```python
from build123d import *

# Parameters (mm, degrees)
SKETCH_1_W      = 84.65
SKETCH_1_H      = 48
SKETCH_1_R      = 1.5
EXTRUDE_1_DEPTH = 1.63
FILLET_1_R      = 3
SKETCH_4_W      = 7.5
SKETCH_4_H      = 8.6
EXTRUDE_2_DEPTH = 27.44
EXTRUDE_3_DEPTH = 16


with BuildPart() as part:
    # 草图1 → 凸台-拉伸1 (new body)
    with BuildSketch(Plane(origin=(0, 0, 0), x_dir=(1, 0, 0), z_dir=(0, 1, 0))):
        with Locations((42.325, 24)):
            Rectangle(SKETCH_1_W, SKETCH_1_H)
        with Locations(Location((2.9, 45, 0), (0, 0, 270))):
            Circle(SKETCH_1_R, mode=Mode.SUBTRACT)
        with Locations(Location((2.9, 13.3, 0), (0, 0, 270))):
            Circle(SKETCH_1_R, mode=Mode.SUBTRACT)
        with Locations(Location((82.15, 45, 0), (0, 0, 270))):
            Circle(SKETCH_1_R, mode=Mode.SUBTRACT)
        with Locations(Location((82.15, 13.3, 0), (0, 0, 270))):
            Circle(SKETCH_1_R, mode=Mode.SUBTRACT)
    extrude(amount=EXTRUDE_1_DEPTH)

    # 圆角1
    fillet_1_edges = [part.edges().sort_by_distance(p)[0] for p in [
        (0, 0.815, 0),
        (0, 0.815, -48),
        (84.65, 0.815, -48),
        (84.65, 0.815, 0),
    ]]
    fillet(fillet_1_edges, radius=FILLET_1_R)

    # 草图4 → 凸台-拉伸2 (add)
    with BuildSketch(Plane(origin=(51.65, 0, 0), x_dir=(0, 0, -1), z_dir=(1, 0, 0))):
        with Locations((3.75, 5.93)):
            Rectangle(SKETCH_4_W, SKETCH_4_H)
    extrude(amount=EXTRUDE_2_DEPTH)

    # 草图5 → 凸台-拉伸3 (add)
    with BuildSketch(Plane(origin=(0, 1.63, 0), x_dir=(1, 0, 0), z_dir=(0, 1, 0))):
        Polygon((62.31, 29.58), (62.31, 16.3), (59.81, 13.98), (58.31, 13.98), (56.81, 13.98), (54.31, 16.3), (54.31, 29.58), align=None)
        Polygon((10.31, 13.98), (8.81, 13.98), (6.31, 16.3), (6.31, 29.58), (14.31, 29.58), (14.31, 16.3), (11.81, 13.98), align=None)
    extrude(amount=EXTRUDE_3_DEPTH)


solid = part.part
```
Build history of the part. All positions in model axes, mm. A direction names the side the tool comes from. Coordinates: 2 decimals unless noted, no trailing zeros. Order: outer loops, then holes, each group sorted by start corner. A loop starts at its lowest first (then second) coordinate and runs counter-clockwise, first axis right, second up.
Item 1: Mould opens along X. For faces 5 (the flat face through (7.58, 9.52, -15.12)), 6 (the flat face through (13.08, 9.52, -15.16)), 7 (the flat face through (10, 10, -13.98)), 8 (the flat face through (61.08, 9.52, -15.16)) say: released by +X, released by -X, zero draft, split by the parting line, or undercut.
Filled in:
face 5: released by -X
face 6: undercut
face 7: zero draft
face 8: released by +X
Item 2: Tool access for faces 1 (the flat face through (6.31, 10, -23)), 2 (the flat face through (14.31, 10, -23)), 3 (the flat face through (65, 6, -7.5)), 4 (the flat face through (54.31, 10, -23)): list every direction of +Z, -Z, +X, -X, +Y, -Y with a clear straight run to the whole face (end or side of a thin tool).
Filled in:
face 1: +Z, -Z, -X, +Y
face 2: +Z, -Z, +Y
face 3: +X, -X, +Y
face 4: -Z, +Y
Item 3: Saw through at A-A on y = 6. List the corners of the cut face in (x, z), then the cut area to 3 significant figures.
Filled in:
outline: (6.31, -29.58) - (14.31, -29.58) - (14.31, -16.3) - (11.81, -13.98) - (8.81, -13.98) - (6.31, -16.3) - close; (51.65, -7.5) - (79.09, -7.5) - (79.09, 0) - (51.65, 0) - close; (54.31, -29.58) - (62.31, -29.58) - (62.31, -16.3) - (59.81, -13.98) - (56.81, -13.98) - (54.31, -16.3) - close
area: 444 mm2
Item 4: Saw through at C-C on x = 65. List the corners of the cut face in (y, z), then the cut area to 3 significant figures.
Filled in:
outline: (0, -48) - (1.63, -48) - (1.63, -7.5) - (10.23, -7.5) - (10.23, 0) - (0, 0) - close
area: 143 mm2
Item 5: Saw through at B-B on y = 13.75. List the corners of the cut face in (x, z).
Filled in:
outline: (6.31, -29.58) - (14.31, -29.58) - (14.31, -16.3) - (11.81, -13.98) - (8.81, -13.98) - (6.31, -16.3) - close; (54.31, -29.58) - (62.31, -29.58) - (62.31, -16.3) - (59.81, -13.98) - (56.81, -13.98) - (54.31, -16.3) - close
Item 6: Drill centre lines: L1, parallel to X at y = 0.6, z = -45; L2, parallel to Z at x = 82.15, y = 0.75; L3, parallel to X at y = 16, z = -28.5. Where is each one in solid material? Low to high.
Filled in:
L1: x = 0 to 1.4, 4.4 to 80.65, 83.65 to 84.65
L2: z = -47.96 to -46.5, -43.5 to -14.8, -11.8 to -0.04
L3: x = 6.31 to 14.31, 54.31 to 62.31
Item 7: Saw through at D-D on z = -10.5. List the corners of the cut face in (x, y), then the cut area to 3 significant figures.
Filled in:
outline: (0, 0) - (84.65, 0) - (84.65, 1.63) - (0, 1.63) - close
area: 138 mm2
Item 8: Drop flat-ended pins along their axis: pin 1 Ø10 at (x, y) = (18, 7.5) entering from +Z; pin 2 Ø8 at (y, z) = (7, -3) entering from -X; pin 3 Ø1 at (x, z) = (20, -36.5) entering from +Y; pin 4 Ø2.5 at (x, z) = (82.15, -13.3) entering from -Y. Give the stop position or say it passes through.
Filled in:
pin 1: stops at z = -15.08
pin 2: stops at x = 51.65
pin 3: stops at y = 1.63
pin 4: passes through
